CAD build for the part. Positions are in the model's coordinates, mm. Face numbers are marked on the shaded views. A direction names the side the tool comes from. Coordinates: 2 decimals unless noted, no trailing zeros. Order: outer loops, then holes, each group sorted by start corner. A loop starts at its lowest first (then second) coordinate and runs counter-clockwise, first axis right, second up. Notation, with made-up numbers: (-33.5, -31) - (-26.5, -31) arc R11 cw to (-26.5, -16) - close; hole circle Ø10 at (-17, 1). An arc over 180 degrees is marked (long way). Write each question's results on one line, items separated by ' | '. Start each with the question number.
Q1. Pull direction Y, two halves, no side cores. Call the marked faces 5, 6, 7 and 8: released by +Y, released by -Y, zero draft, split by the parting line, or undercut.
Q2. Wall check: probe 1 along X at (y, z) = (-0.5, 1.75); probe 2 along Y at (x, z) = (42.4, 1); probe 3 along Z at (x, y) = (42, -55.5). Give the ranges that are in metal, low to high.
Q3. Band-saw the part on D-D, the plane y = -12. Write the cut outline in (x, z).
Q4. Band-saw the part on C-C, the plane z = -8. Write the cut outline in (x, y), then the cut area to 4 significant figures.
Q5. Which spindle directions (+Z, -Z, +X, -X, +Y, -Y) get a long thin tool onto all of the face, cutting with end or side? Do the marked faces 1, 2, 3 and 4. Say none if no direction does.
Q6. Band-saw the part on A-A, the plane y = -3. Write the cut outline in (x, z).
Q7. Band-saw the part on B-B, the plane y = -31.8. Write the cut outline in (x, z), then the cut area to 3 significant figures.
Q8. Pin check, flat tips, straight feed: P1, Ø1.1, axis at x = 49, y = -64.5, coming from the -Z side; P2, Ø4, axis at x = 39, z = 0, coming from the -Y side; P3, Ø0.5, axis at x = 35, y = 0.5, coming from the +Z side. Stop position of each tip, or through.
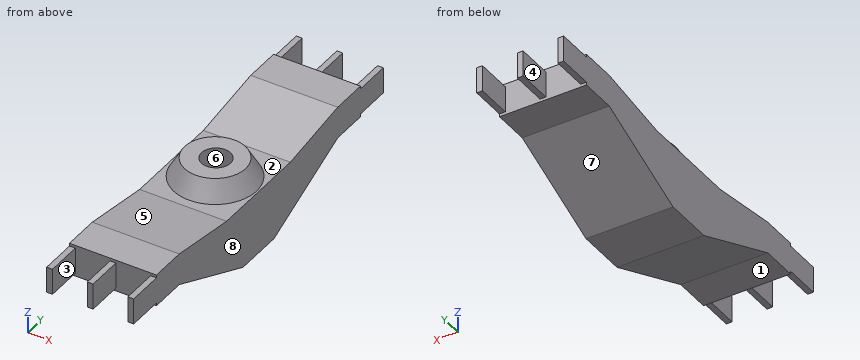
```python
from build123d import *

# Parameters (mm, degrees)
CYLINDER_R                 = 2.5
CYLINDER_DEPTH             = 6
EXTRUDE024_DEPTH           = 6
EXTRUDE024_PLACEMENT_ANGLE = 90
EXTRUDE023_DEPTH           = 1
EXTRUDE023_PLACEMENT_ANGLE = 90
EXTRUDE025_DEPTH           = 6
EXTRUDE025_PLACEMENT_ANGLE = 90
EXTRUDE_DEPTH              = 1
EXTRUDE_PLACEMENT_ANGLE    = 90
REVOLVE_PLACEMENT_ANGLE    = 90
EXTRUDE022_DEPTH           = 1
EXTRUDE022_PLACEMENT_ANGLE = 90


with BuildPart() as cylinder:
    # Cylinder → Cylinder (new body)
    with BuildSketch(Plane(origin=(42.4, -33.3, -0.5), x_dir=(1, 0, 0), z_dir=(0, 0, 1))):
        Circle(CYLINDER_R)
    extrude(amount=CYLINDER_DEPTH)


with BuildPart() as extrude024:
    # Sketch016 → Extrude024 (new body)
    with BuildSketch(Plane.YZ):
        Polygon((5.5, -12.57), (3.5, -25.57), (3.5, -43.07), (5.5, -56.07), (5.5, -62.32), (0, -62.32), (0, -56.07), (-7.5, -38.57), (-7.5, -30.07), (0, -12.57), (0, -6.32), (5.5, -6.32), align=None)
    extrude(amount=EXTRUDE024_DEPTH)


with BuildPart() as extrude024_1:
    # Extrude024 placement: moved
    add(extrude024.part.moved(Location((35.7, -67.57, -2.3))).rotate(Axis((35.7, -67.57, -2.3), (1, 0, 0)), EXTRUDE024_PLACEMENT_ANGLE))


with BuildPart() as extrude023:
    # Sketch002 → Extrude023 (new body)
    with BuildSketch(Plane.XY):
        Polygon((5.5, -12.5), (3.5, -25.5), (3.5, -43), (5.5, -56), (5.5, -62.25), (5, -62.25), (5, -68.5), (0.5, -68.5), (0.5, -62.25), (0, -62.25), (0, -56), (-7.5, -38.5), (-7.5, -30), (0, -12.5), (0, -6.25), (0.5, -6.25), (0.5, 0), (5, 0), (5, -6.25), (5.5, -6.25), align=None)
    extrude(amount=EXTRUDE023_DEPTH)


with BuildPart() as extrude023_1:
    # Extrude023 placement: moved
    add(extrude023.part.moved(Location((42.7, 1, -2.3))).rotate(Axis((42.7, 1, -2.3), (0, -1, 0)), EXTRUDE023_PLACEMENT_ANGLE))


with BuildPart() as extrude025:
    # Sketch016 → Extrude025 (new body)
    with BuildSketch(Plane.YZ):
        Polygon((5.5, -12.57), (3.5, -25.57), (3.5, -43.07), (5.5, -56.07), (5.5, -62.32), (0, -62.32), (0, -56.07), (-7.5, -38.57), (-7.5, -30.07), (0, -12.57), (0, -6.32), (5.5, -6.32), align=None)
    extrude(amount=EXTRUDE025_DEPTH)


with BuildPart() as extrude025_1:
    # Extrude025 placement: moved
    add(extrude025.part.moved(Location((42.7, -67.57, -2.3))).rotate(Axis((42.7, -67.57, -2.3), (1, 0, 0)), EXTRUDE025_PLACEMENT_ANGLE))


with BuildPart() as extrude_body:
    # Sketch002 → Extrude (new body)
    with BuildSketch(Plane.XY):
        Polygon((5.5, -12.5), (3.5, -25.5), (3.5, -43), (5.5, -56), (5.5, -62.25), (5, -62.25), (5, -68.5), (0.5, -68.5), (0.5, -62.25), (0, -62.25), (0, -56), (-7.5, -38.5), (-7.5, -30), (0, -12.5), (0, -6.25), (0.5, -6.25), (0.5, 0), (5, 0), (5, -6.25), (5.5, -6.25), align=None)
    extrude(amount=EXTRUDE_DEPTH)


with BuildPart() as extrude_body_1:
    # Extrude placement: moved
    add(extrude_body.part.moved(Location((49.7, 1, -2.3))).rotate(Axis((49.7, 1, -2.3), (0, -1, 0)), EXTRUDE_PLACEMENT_ANGLE))


with BuildPart() as revolve_body:
    # Sketch003 → Revolve (revolve)
    with BuildSketch(Plane.XZ):
        Polygon((1.919868, -28.090362), (1.919868, -35.340362), (5.419868, -35.340362), (5.419868, -30.090362), align=None)
    revolve(axis=Axis((5.419868, 0, -35.340362), (1, 0, 0)))


with BuildPart() as revolve_body_1:
    # Revolve placement: moved
    add(revolve_body.part.moved(Location((6.9, -33.3, -0.9))).rotate(Axis((6.9, -33.3, -0.9), (0, -1, 0)), REVOLVE_PLACEMENT_ANGLE))


with BuildPart() as obj1:
    # Sketch002 → Extrude022 (new body)
    with BuildSketch(Plane.XY):
        Polygon((5.5, -12.5), (3.5, -25.5), (3.5, -43), (5.5, -56), (5.5, -62.25), (5, -62.25), (5, -68.5), (0.5, -68.5), (0.5, -62.25), (0, -62.25), (0, -56), (-7.5, -38.5), (-7.5, -30), (0, -12.5), (0, -6.25), (0.5, -6.25), (0.5, 0), (5, 0), (5, -6.25), (5.5, -6.25), align=None)
    extrude(amount=EXTRUDE022_DEPTH)


with BuildPart() as obj1_1:
    # Extrude022 placement: moved
    add(obj1.part.moved(Location((35.7, 1, -2.3))).rotate(Axis((35.7, 1, -2.3), (0, -1, 0)), EXTRUDE022_PLACEMENT_ANGLE))

    # Fusion: union Revolve body
    add(revolve_body_1.part)

    # Fusion057: union Extrude024, Extrude023, Extrude025, Extrude body
    add(extrude024_1.part)
    add(extrude023_1.part)
    add(extrude025_1.part)
    add(extrude_body_1.part)

    # Cut064: cut Cylinder
    add(cylinder.part, mode=Mode.SUBTRACT)


with BuildPart() as obj1_2:
    # Cut064 placement: moved
    add(obj1_1.part.moved(Location((0, 1.5, 0))))


solid = obj1_2.part
```
Results below:
1) face 5: undercut | face 6: undercut | face 7: released by +Y | face 8: zero draft
2) probe 1: x = 34.7 to 35.7, 41.7 to 42.7, 48.7 to 49.7 | probe 2: y = -66 to -34.3, -29.3 to 2.5 | probe 3: z = -2.3 to 3.2
3) outline: (34.7, -3.16) - (49.7, -3.16) - (49.7, 2.89) - (34.7, 2.89) - close
4) outline: (34.7, -40.2) - (49.7, -40.2) - (49.7, -23.3) - (34.7, -23.3) - close | area: 253.5 mm²
5) face 1: -Z, +X, -X, -Y | face 2: +Z | face 3: +Z, -Z, -Y | face 4: +Z, -Z, +Y
6) outline: (34.7, -1.8) - (35.7, -1.8) - (35.7, 2.7) - (34.7, 2.7) - close; (41.7, -1.8) - (42.7, -1.8) - (42.7, 2.7) - (41.7, 2.7) - close; (48.7, -1.8) - (49.7, -1.8) - (49.7, 2.7) - (48.7, 2.7) - close
7) outline: (34.7, -9.8) - (49.7, -9.8) - (49.7, 1.2) - (49.39, 1.2) - (47.49, 4.52) - (44.9, 4.52) - (44.9, -0.5) - (39.9, -0.5) - (39.9, 4.52) - (36.99, 4.52) - (35.09, 1.2) - (34.7, 1.2) - close | area: 181 mm²
8) P1: stops at z = -1.8 | P2: stops at y = -59.75 | P3: stops at z = 2.7
